from build123d import *

# Parameters (mm, degrees)
BOSS_EXTRUDE1_DEPTH = 6.35
FILLET1_R           = 6.35
FILLET2_R           = 76.2


with BuildPart() as part:
    # Sketch1 → Boss-Extrude1 (new body)
    with BuildSketch(Plane(origin=(0, 0, 0), x_dir=(1, 0, 0), z_dir=(0, 1, 0))):
        Polygon((0, 0), (0, 228.6), (-323.85, 228.6), (-323.85, 203.2), (-25.4, 203.2), (-25.4, 0), align=None)
    extrude(amount=BOSS_EXTRUDE1_DEPTH)

    # Fillet1
    fillet1_edges = [part.edges().sort_by_distance(p)[0] for p in [
        (-25.4, 3.175, 0),
        (-323.85, 3.175, -203.2),
        (-323.85, 3.175, -228.6),
        (0, 3.175, -228.6),
        (0, 3.175, 0),
    ]]
    fillet(fillet1_edges, radius=FILLET1_R)

    # Fillet2
    fillet2_edges = [part.edges().sort_by_distance(p)[0] for p in [
        (-25.4, 3.175, -203.2),
    ]]
    fillet(fillet2_edges, radius=FILLET2_R)


solid = part.part
CAD build for the part. Positions are in the model's coordinates, mm. A direction names the side the tool comes from. Give positions to 0.01 mm unless a question says otherwise; leave off trailing zeros. Order: outer loops, then holes, each group sorted by start corner. A loop starts at its lowest first (then second) coordinate and runs counter-clockwise, first axis right, second up. Notation, with made-up numbers: (10, 86.5) - (65, 86.5) arc R18 ccw to (65, 115.5) - close; hole circle Ø7 at (46, 82). An arc over 180 degrees is marked (long way). Answer in a Markdown table with one row per item.
1. Saw through at C-C, the plane x = -262. Give the cut face in (y, z), plus the area to 3 significant figures.
Data:
| item | result |
|---|---|
| outline | (0, -228.6) - (6.35, -228.6) - (6.35, -203.2) - (0, -203.2) - close |
| area | 161 mm² |
2. Saw through at B-B, the plane z = -122.5. Give the cut face in (x, y), plus the area to 3 significant figures.
Data:
| item | result |
|---|---|
| outline | (-25.4, 0) - (0, 0) - (0, 6.35) - (-25.4, 6.35) - close |
| area | 161 mm² |
3. Flat gauge pins, fed straight in: pin 1 (1.5 mm diameter, centred on y = 5, z = -176.5, fed in from -X); pin 2 (3 mm diameter, centred on y = 4.5, z = -83, fed in from -X); pin 3 (3 mm diameter, centred on x = -253, y = 2.5, fed in from +Z). Where does each tip first touch, or does it go through?
Data:
| item | result |
|---|---|
| pin 1 | stops at x = -44.32 |
| pin 2 | stops at x = -25.4 |
| pin 3 | stops at z = -203.2 |
4. Probe probe 1 along X at (y, z) = (1.75, -88.5); probe 2 along Z at (x, y) = (-244, 2); probe 3 along X at (y, z) = (5.75, -134.5). List the from-to ranges inside material, lowest first. Write a range as [from, to].
Data:
| item | result |
|---|---|
| probe 1 | x = [-25.4, 0] |
| probe 2 | z = [-228.6, -203.2] |
| probe 3 | x = [-25.77, 0] |
5. Tool access for faces 1 (the flat face through (-115, 0, -208)), 2 (the flat face through (-211, 3, -203.2)): list every direction of +Z, -Z, +X, -X, +Y, -Y with a clear straight run to the whole face (end or side of a thin tool).
Data:
| item | result |
|---|---|
| face 1 | +Z, -Z, +X, -X, -Y |
| face 2 | +Z, -X, +Y, -Y |
6. Saw through at A-A, the plane y = 1. Give the cut face in (x, z), plus the area to 3 significant figures.
Data:
| item | result |
|---|---|
| outline | (-323.85, -222.25) arc R6.35 ccw to (-317.5, -228.6) - (-6.35, -228.6) arc R6.35 ccw to (0, -222.25) - (0, -6.35) arc R6.35 ccw to (-6.35, 0) - (-19.05, 0) arc R6.35 ccw to (-25.4, -6.35) - (-25.4, -127) arc R76.2 cw to (-101.6, -203.2) - (-317.5, -203.2) arc R6.35 ccw to (-323.85, -209.55) - close |
| area | 14,600 mm² |
